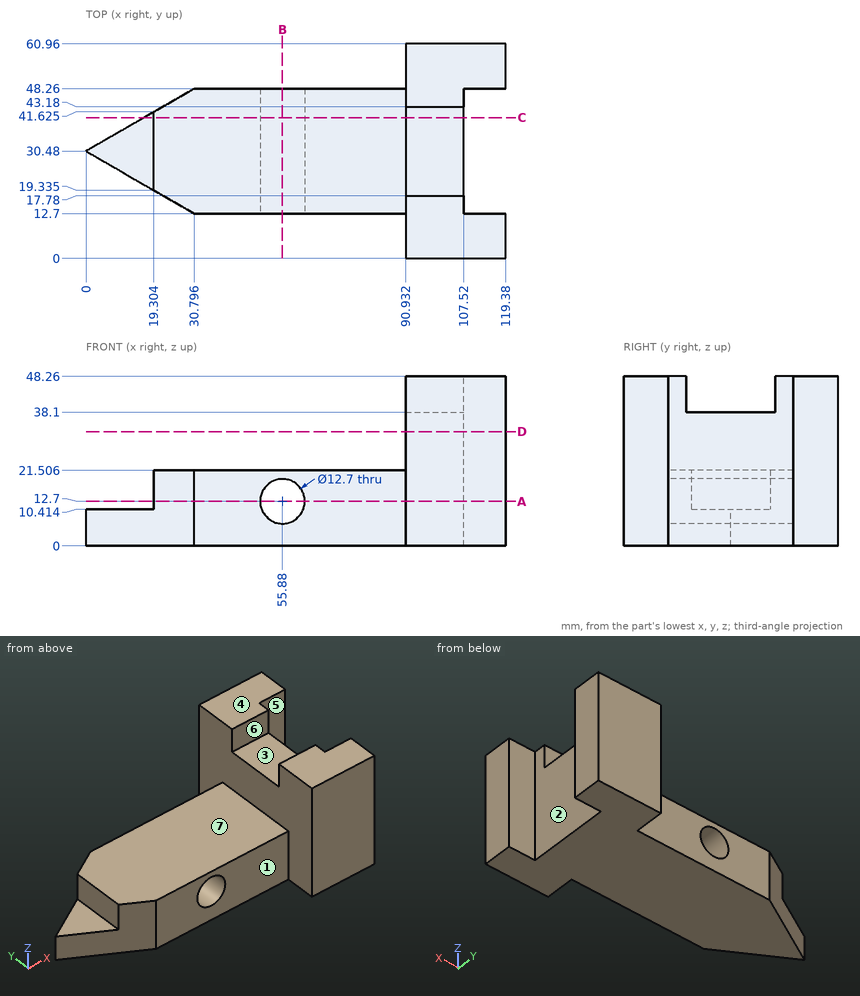
Print and shaded views of the part. All mm, measured from the part's lowest x, y and z. A direction names the side the tool comes from. Round coordinates to 2 decimals unless told otherwise and drop trailing zeros. Write each loop counter-clockwise with the first axis right and the second up, starting at its lowest first coordinate (ties: lowest second). Pieces come first, ordered by that corner, then holes. Notation, with made-up numbers: M 5,71.5 L 62,71.5 A22 ccw 62,79.5 Z; hole C 48.5,76.25 d9. An arc over 180 degrees is marked long. Use a Markdown table: item, result. Add a question column.
1. Slice it at D-D on z = 32.5. Give the cut face in (x, y).
2. 3-axis set-ups, long thin cutter, end or side, ignore diameter. For the marked faces 5, 6 and 7: which of +Z, -Z, +X, -X, +Y, -Y reach the whole face in a straight line?
3. Slice it at A-A on z = 12.7. Give the cut face in (x, y) (1 decimal), then the cut area to 3 significant figures.
4. Slice it at C-C on y = 40. Give the cut face in (x, z), then the cut area to 4 significant figures.
5. Drill centre lines: probe 1 along Y at (x, z) = (111.5, 38); probe 2 along Z at (x, y) = (55.88, 31.5); probe 3 along X at (y, z) = (53.5, 13.5). Where is each one in solid material? Low to high.
6. Slice it at B-B on x = 55.88. Give the cut face in (y, z).
7. Pull direction Y, two halves, no side cores. Call the marked faces 1, 2, 3 and 4: released by +Y, released by -Y, zero draft, split by the parting line, or undercut.
8. Flat gauge pins, fed straight in: P1, Ø3.5, axis at y = 25.5, z = 16.5, coming from the -X side; P2, Ø15.5, axis at x = 10.5, y = 33.5, coming from the +Z side; P3, Ø4, axis at y = 45.5, z = 21.5, coming from the +X side; P4, Ø6.5, axis at x = 55.5, z = 11.5, coming from the +Y side (3 decimals). Where does each tip first touch, or does it go through?
Reply:
| question | item | result |
|---|---|---|
| 1 | outline | M 90.93,0 L 119.38,0 L 119.38,12.7 L 107.52,12.7 L 107.52,48.26 L 119.38,48.26 L 119.38,60.96 L 90.93,60.96 Z |
| 2 | face 5 | +Z, -Z, +X |
| 2 | face 6 | +Z, +X, -X |
| 2 | face 7 | +Z, -X, +Y, -Y |
| 3 | outline | M 19.3,19.3 L 30.8,12.7 L 49.5,12.7 L 49.5,48.3 L 30.8,48.3 L 19.3,41.6 Z; M 62.2,12.7 L 90.9,12.7 L 90.9,0 L 119.4,0 L 119.4,12.7 L 107.5,12.7 L 107.5,48.3 L 119.4,48.3 L 119.4,61 L 90.9,61 L 90.9,48.3 L 62.2,48.3 Z |
| 3 | area | 3,330 mm^2 |
| 4 | outline | M 16.49,0 L 107.52,0 L 107.52,38.1 L 90.93,38.1 L 90.93,21.51 L 19.3,21.51 L 19.3,10.41 L 16.49,10.41 Z; hole C 55.88,12.7 d12.7 |
| 4 | area | 2,075 mm^2 |
| 5 | probe 1 | y = 0 to 12.7, 48.26 to 60.96 |
| 5 | probe 2 | z = 0 to 6.35, 19.05 to 21.51 |
| 5 | probe 3 | x = 90.93 to 119.38 |
| 6 | outline | M 12.7,0 L 48.26,0 L 48.26,6.35 L 12.7,6.35 Z; M 12.7,19.05 L 48.26,19.05 L 48.26,21.51 L 12.7,21.51 Z |
| 7 | face 1 | released by -Y |
| 7 | face 2 | undercut |
| 7 | face 3 | undercut |
| 7 | face 4 | zero draft |
| 8 | P1 | stops at x = 19.3 |
| 8 | P2 | stops at z = 10.41 |
| 8 | P3 | stops at x = 107.52 |
| 8 | P4 | passes through |
